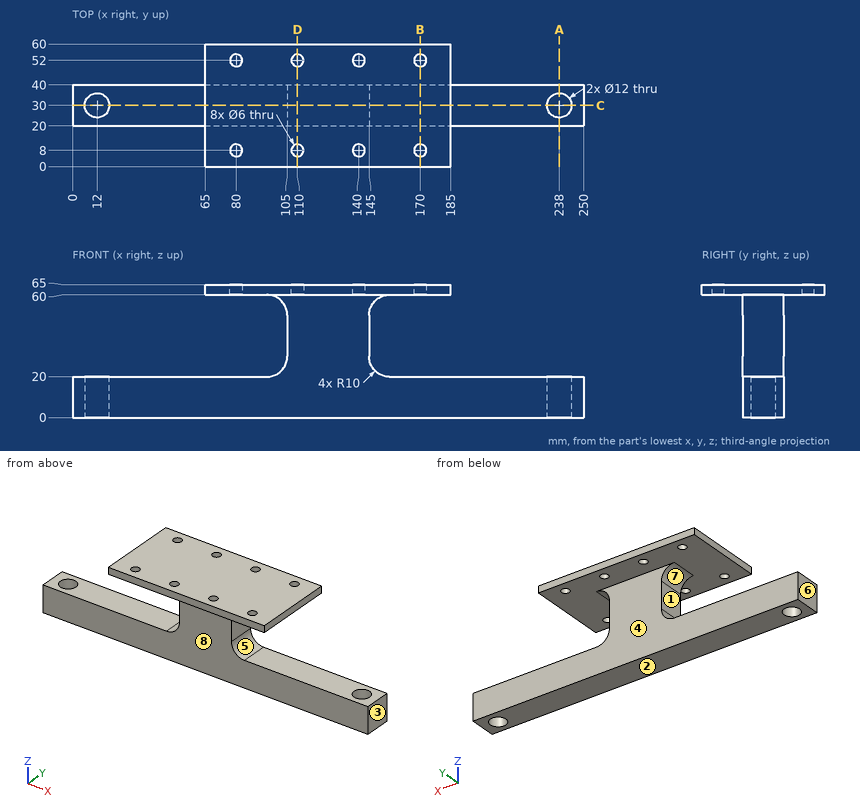
Part print with two shaded views. Sizes in mm from the minimum x, y, z corner. A direction names the side the tool comes from. Coordinates: 2 decimals unless noted, no trailing zeros. Order: outer loops, then holes, each group sorted by start corner. A loop starts at its lowest first (then second) coordinate and runs counter-clockwise, first axis right, second up.
(1) Drill centre lines: L1, parallel to Y at x = 80, z = 63.65; L2, parallel to Y at x = 12, z = 5; L3, parallel to X at y = 32, z = 12.5. Where is each one in solid material? Low to high.
Solution:
L1: y = 0 to 5, 11 to 49, 55 to 60
L2: y = 20 to 24, 36 to 40
L3: x = 0 to 6.34, 17.66 to 232.34, 243.66 to 250
(2) Saw through at D-D, the plane x = 110. Write the cut outline in (y, z).
Solution:
outline: (0, 60) - (5, 60) - (5, 65) - (0, 65) - close; (11, 60) - (20, 60) - (20, 0) - (40, 0) - (40, 60) - (49, 60) - (49, 65) - (11, 65) - close; (55, 60) - (60, 60) - (60, 65) - (55, 65) - close
(3) Saw through at A-A, the plane x = 238. Write the cut outline in (y, z).
Solution:
outline: (20, 0) - (24, 0) - (24, 20) - (20, 20) - close; (36, 0) - (40, 0) - (40, 20) - (36, 20) - close
(4) Saw through at C-C, the plane y = 30. Write the cut outline in (x, z), and give its area (3 significant figures).
Solution:
outline: (0, 0) - (6, 0) - (6, 20) - (0, 20) - close; (18, 0) - (232, 0) - (232, 20) - (155, 20) arc R10 cw to (145, 30) - (145, 50) arc R10 cw to (155, 60) - (185, 60) - (185, 65) - (65, 65) - (65, 60) - (95, 60) arc R10 cw to (105, 50) - (105, 30) arc R10 cw to (95, 20) - (18, 20) - close; (244, 0) - (250, 0) - (250, 20) - (244, 20) - close
area: 6,810 mm2
(5) Which spindle directions (+Z, -Z, +X, -X, +Y, -Y) get a long thin tool onto all of the face, cutting with end or side? Do the marked faces 4, 5, 6, 7 and 8. Say none if no direction does.
Solution:
face 4: -Z, +X, -X, +Y
face 5: +X, +Y, -Y
face 6: +Z, -Z, -X, +Y, -Y
face 7: -X, +Y, -Y
face 8: -Z, +X, -X, -Y
(6) Pin check, flat tips, straight feed: pin 1 Ø9.5 at (x, y) = (110, 52) entering from -Z; pin 2 Ø12 at (x, z) = (72, 17.5) entering from -Y; pin 3 Ø5.5 at (y, z) = (20.5, 62) entering from -X. Stop position of each tip, or through.
Solution:
pin 1: stops at z = 60
pin 2: stops at y = 20
pin 3: stops at x = 65
(7) Saw through at B-B, the plane x = 170. Write the cut outline in (y, z).
Solution:
outline: (0, 60) - (5, 60) - (5, 65) - (0, 65) - close; (11, 60) - (49, 60) - (49, 65) - (11, 65) - close; (20, 0) - (40, 0) - (40, 20) - (20, 20) - close; (55, 60) - (60, 60) - (60, 65) - (55, 65) - close
(8) Mould opens along Z. For the marked faces 1, 2 and 3 say: released by +Z, released by -Z, zero draft, split by the parting line, or undercut.
Solution:
face 1: undercut
face 2: released by -Z
face 3: zero draft
